Here's how the part is built. I have some questions about the finished solid (model axes, mm). A direction names the side the tool comes from. Coordinates: 2 decimals unless noted, no trailing zeros. Loops run counter-clockwise (first coordinate to the right, second up) from the corner with the lowest first, then second, coordinate; pieces in that order, holes last. Notation, with made-up numbers: (-4, -1.75) -> (21, -1.75) arc R17 ccw to (21, 19.25) -> close; hole circle Ø1 at (-6, 69.25). An arc over 180 degrees is marked (long way). Answer as a JSON object with one key per item and string values. Group by question number.
Q1. On a 3-axis mill with a long thin cutter (end or side, diameter ignored), from which of +Z, -Z, +X, -X, +Y, -Y can I reach the whole of each face in a straight line? I mean faces 1 (the flat face through (8, 1, 0)), 2 (the cylindrical face through (-0.325, 0.507, -8.536)). Say none if no direction works.
Q2. I need wall thicknesses on line 1 (Z direction, x = 0, y = 0.3); line 2 (X direction, y = 1.95, z = 0); line 3 (X direction, y = 1.65, z = 0). Which ranges of each line are inside material? Lowest first, please.
Q3. I'm going to push flat-ended pins straight in: pin 1 (5.5 mm diameter, centred on x = -1, z = 9.5, fed in from +Y); pin 2 (2.5 mm diameter, centred on x = 11, z = 0, fed in from +Y); pin 3 (4 mm diameter, centred on x = -3.5, z = 1.5, fed in from +Y). Where does each tip first touch, or does it pass through?
Q4. I want a section at A-A on z = 0. Write out the boundary of the cut face in (x, y).
Q5. Thinking about a two-plate mould opening in Z: for faces 3 (the flat face through (3, 2.5, 3)), 4 (the cylindrical face through (8.536, 0.507, -0.325)), 5 (the cylindrical face through (-0.29, 6.47, 1.32)), which applies, released by +Z, released by -Z, zero draft, split by the parting line, or undercut?
Q6. I want a section at B-B on x = 0. Write out the boundary of the cut face in (y, z).
Q7. I want a section at C-C on y = 6. Write out the boundary of the cut face in (x, z), then the cut area to 3 significant figures.
```python
from build123d import *

# Parameters (mm, degrees)
SKETCH1_R           = 15
BOSS_EXTRUDE1_DEPTH = 2.5
SKETCH2_R           = 1.5
CUT_EXTRUDE1_DEPTH  = 3.5
SKETCH4_R           = 2.5
CUT_EXTRUDE2_DEPTH  = 1.5
CIRPATTERN1_COUNT   = 4
SKETCH3_R           = 1.35
BOSS_EXTRUDE2_DEPTH = 6
FILLET2_R           = 2
FILLET3_R           = 2


with BuildPart() as part:
    # Sketch1 → Boss-Extrude1 (new body)
    with BuildSketch(Plane(origin=(0, 0, 0), x_dir=(1, 0, 0), z_dir=(0, 1, 0))):
        Circle(SKETCH1_R)
    extrude(amount=BOSS_EXTRUDE1_DEPTH)

    # Sketch2 → Cut-Extrude1 (cut, through all)
    with BuildSketch(Plane(origin=(0, 2.5, 0), x_dir=(1, 0, 0), z_dir=(0, 1, 0))):
        with Locations((0, 10)):
            Circle(SKETCH2_R)
    cut_extrude1 = extrude(amount=-CUT_EXTRUDE1_DEPTH, mode=Mode.SUBTRACT)

    # Sketch4 → Cut-Extrude2 (cut)
    with BuildSketch(Plane(origin=(0, 2.5, 0), x_dir=(1, 0, 0), z_dir=(0, 1, 0))):
        with Locations((0, 10)):
            Circle(SKETCH4_R)
    cut_extrude2 = extrude(amount=-CUT_EXTRUDE2_DEPTH, mode=Mode.SUBTRACT)

    # CirPattern1: Cut-Extrude1, Cut-Extrude2 ×4 about axis
    cirpattern1_axis = Axis((0, 0, 0), (0, 1, 0))
    for i in range(1, CIRPATTERN1_COUNT):
        add(cut_extrude1.rotate(cirpattern1_axis, i * 360 / CIRPATTERN1_COUNT), mode=Mode.SUBTRACT)
        add(cut_extrude2.rotate(cirpattern1_axis, i * 360 / CIRPATTERN1_COUNT), mode=Mode.SUBTRACT)

    # Sketch3 → Boss-Extrude2 (add)
    with BuildSketch(Plane(origin=(0, 2.5, 0), x_dir=(1, 0, 0), z_dir=(0, 1, 0))):
        Circle(SKETCH3_R)
    extrude(amount=BOSS_EXTRUDE2_DEPTH)

    # Fillet2
    fillet2_edges = [part.edges().sort_by_distance(p)[0] for p in [
        (-1.35, 2.5, 0),
    ]]
    fillet(fillet2_edges, radius=FILLET2_R)

    # Fillet3
    fillet3_edges = [part.edges().sort_by_distance(p)[0] for p in [
        (-15, 2.5, 0),
    ]]
    fillet(fillet3_edges, radius=FILLET3_R)


solid = part.part
```
Result set:
{
 "1": {"face 1": "+Y", "face 2": "+Y, -Y"},
 "2": {"line 1": "z = -15 to -11.5, -8.5 to 8.5, 11.5 to 15", "line 2": "x = -14.38 to -12.5, -7.5 to 7.5, 12.5 to 14.38", "line 3": "x = -14.64 to -12.5, -7.5 to 7.5, 12.5 to 14.64"},
 "3": {"pin 1": "stops at y = 2.5", "pin 2": "stops at y = 1", "pin 3": "stops at y = 3.23"},
 "4": {"outline": "(-15, 0) -> (-11.5, 0) -> (-11.5, 1) -> (-12.5, 1) -> (-12.5, 2.5) -> (-13, 2.5) arc R2 ccw to (-15, 0.5) -> close; (-8.5, 0) -> (8.5, 0) -> (8.5, 1) -> (7.5, 1) -> (7.5, 2.5) -> (3.35, 2.5) arc R2 cw to (1.35, 4.5) -> (1.35, 8.5) -> (-1.35, 8.5) -> (-1.35, 4.5) arc R2 cw to (-3.35, 2.5) -> (-7.5, 2.5) -> (-7.5, 1) -> (-8.5, 1) -> close; (11.5, 0) -> (15, 0) -> (15, 0.5) arc R2 ccw to (13, 2.5) -> (12.5, 2.5) -> (12.5, 1) -> (11.5, 1) -> close"},
 "5": {"face 3": "zero draft", "face 4": "undercut", "face 5": "split by the parting line"},
 "6": {"outline": "(0, -15) -> (0.5, -15) arc R2 ccw to (2.5, -13) -> (2.5, -12.5) -> (1, -12.5) -> (1, -11.5) -> (0, -11.5) -> close; (0, -8.5) -> (1, -8.5) -> (1, -7.5) -> (2.5, -7.5) -> (2.5, -3.35) arc R2 cw to (4.5, -1.35) -> (8.5, -1.35) -> (8.5, 1.35) -> (4.5, 1.35) arc R2 cw to (2.5, 3.35) -> (2.5, 7.5) -> (1, 7.5) -> (1, 8.5) -> (0, 8.5) -> close; (0, 11.5) -> (1, 11.5) -> (1, 12.5) -> (2.5, 12.5) -> (2.5, 13) arc R2 ccw to (0.5, 15) -> (0, 15) -> close"},
 "7": {"outline": "circle Ø2.7 at (0, 0)", "area": "5.73 mm²"}
}
